Check sheet for the modelled part. Datum: model origin and axes. Units: mm. Face numbers are marked on the shaded views. A direction names the side the tool comes from. Coordinates: 2 decimals unless noted, no trailing zeros. Loops run counter-clockwise (first coordinate to the right, second up) from the corner with the lowest first, then second, coordinate; pieces in that order, holes last. Notation, with made-up numbers: (20.25, 14) - (33.25, 14) arc R25 cw to (33.25, 33) - close; hole circle Ø1 at (-33.5, -8). An arc over 180 degrees is marked (long way). Write each question's results on one line, items separated by ' | '. Start each with the question number.
1. Cross-section at A-A (z = -13). Record the cut outline in (x, y), and give its area (3 significant figures).
2. Cross-section at B-B (y = -170.5). Record the cut outline in (x, z), and give its area (3 significant figures).
3. Tool access check on the marked faces 1 and 2. Record the directions out of +Z, -Z, +X, -X, +Y, -Y that give a thin tool (end or side, any length) a straight path to the whole face; none if there is none.
4. Thickness scan on line 1 (Y direction, x = 11, z = -2.5); line 2 (Z direction, x = -0.5, y = -24); line 3 (Z direction, x = 0.5, y = -146). Record the ranges inside material, lowest first. Write a range as [from, to].
5. Cross-section at D-D (y = -12.5). Record the cut outline in (x, z) (3 decimals), and give its area (3 significant figures).
6. Gauge pin test, flat ends, axial feed: P1, Ø1.9, axis at x = -1, y = -159, coming from the +Z side; P2, Ø12, axis at y = -153, z = 2.5, coming from the -X side; P3, Ø1.5, axis at x = 11.5, y = -89, coming from the -Z side. Record the tip position at first contact, or that the pin passes through.
7. Cross-section at C-C (x = 13). Record the cut outline in (y, z).
```python
from build123d import *

# Parameters (mm, degrees)
CUT_EXTRUDE1_DEPTH      = 286.633670547
CUT_EXTRUDE1_DEPTH_BACK = 286.633670547
CUT_EXTRUDE2_DEPTH      = 286.633670547
CUT_EXTRUDE2_DEPTH_BACK = 286.633670547
BOSS_EXTRUDE1_DEPTH     = 13.7
SKETCH7_W               = 0.1
SKETCH7_H               = 0.8


with BuildPart() as part:
    # Sketch1 → Revolve1 (revolve)
    with BuildSketch(Plane.XY):
        with BuildLine():
            Line((0, 0), (15.875, 0))
            Line((15.875, 0), (15.875, -95.25))
            Line((15.875, -95.25), (7.75, -95.25))
            ThreePointArc((7.75, -95.25), (6.710108543, -97.13103799), (6.35, -99.25))
            Line((6.35, -99.25), (6.35, -123.35))
            ThreePointArc((6.35, -123.35), (6.765423592, -125.271598049), (7.9375, -126.85))
            Line((7.9375, -126.85), (7.9375, -148.15))
            Line((7.9375, -148.15), (6.35, -148.15))
            Line((6.35, -148.15), (6.35, -192.25))
            ThreePointArc((6.35, -192.25), (4.060973326, -193.504085038), (3.15, -195.95))
            Line((3.15, -195.95), (3.15, -236.95))
            ThreePointArc((3.15, -236.95), (2.021186638, -237.921495537), (1.6, -239.35))
            Line((1.6, -239.35), (1.6, -284.75))
            Line((1.6, -284.75), (0, -284.75))
            Line((0, -284.75), (0, 0))
        make_face()
    revolve(axis=Axis((0, -284.75, 0), (0, 1, 0)))

    # Sketch3 → Cut-Extrude1 (cut, two sides: drawn at the far end of the back side and taken through both)
    with BuildSketch(Plane.XY.offset(-CUT_EXTRUDE1_DEPTH_BACK)):
        with BuildLine():
            Line((7.9375, -139.15), (7.9375, -126.85))
            ThreePointArc((7.9375, -126.85), (7.511434792, -126.425239776), (7.14375, -125.949045798))
            Line((7.14375, -125.949045798), (7.14375, -139.15))
            Line((7.14375, -139.15), (7.9375, -139.15))
        make_face()
        with BuildLine():
            Line((-7.14375, -139.15), (-7.14375, -125.949045798))
            ThreePointArc((-7.14375, -125.949045798), (-7.511434792, -126.425239776), (-7.9375, -126.85))
            Line((-7.9375, -126.85), (-7.9375, -139.15))
            Line((-7.9375, -139.15), (-7.14375, -139.15))
        make_face()
    extrude(amount=CUT_EXTRUDE1_DEPTH + CUT_EXTRUDE1_DEPTH_BACK, mode=Mode.SUBTRACT)

    # Sketch4 → Cut-Extrude2 (cut, two sides: drawn at the far end of the back side and taken through both)
    with BuildSketch(Plane(origin=(0, 0, 0), x_dir=(0, 0, -1), z_dir=(1, 0, 0)).offset(-CUT_EXTRUDE2_DEPTH_BACK)):
        with BuildLine():
            Line((6.35, -163.5805), (6.2245, -163.5805))
            ThreePointArc((6.2245, -163.5805), (5.729525253, -163.375474747), (5.5245, -162.8805))
            Line((5.5245, -162.8805), (5.5245, -154.8825))
            ThreePointArc((5.5245, -154.8825), (5.729525253, -154.387525253), (6.2245, -154.1825))
            Line((6.2245, -154.1825), (6.35, -154.1825))
            Line((6.35, -154.1825), (6.35, -163.5805))
        make_face()
        with BuildLine():
            Line((-5.5245, -162.8805), (-5.5245, -154.8825))
            ThreePointArc((-5.5245, -154.8825), (-5.729525253, -154.387525253), (-6.2245, -154.1825))
            Line((-6.2245, -154.1825), (-6.35, -154.1825))
            Line((-6.35, -154.1825), (-6.35, -163.5805))
            Line((-6.35, -163.5805), (-6.2245, -163.5805))
            ThreePointArc((-6.2245, -163.5805), (-5.729525253, -163.375474747), (-5.5245, -162.8805))
        make_face()
    extrude(amount=CUT_EXTRUDE2_DEPTH + CUT_EXTRUDE2_DEPTH_BACK, mode=Mode.SUBTRACT)

    # Sketch5 → Boss-Extrude1 (add)
    with BuildSketch(Plane(origin=(0, 0, 0), x_dir=(1, 0, 0), z_dir=(0, 1, 0))):
        Polygon((-4.33708409, 7.51205), (-8.674168179, 0), (-4.33708409, -7.51205), (4.33708409, -7.51205), (8.674168179, 0), (4.33708409, 7.51205), align=None)
    extrude(amount=BOSS_EXTRUDE1_DEPTH)

    # Sketch6 → Revolve2 (revolve)
    with BuildSketch(Plane.XY, mode=Mode.PRIVATE) as revolve2_sk:
        Polygon((7.35, 13.7), (0, 13.7), (0, 50.2), (5.65, 50.2), align=None)
    revolve(revolve2_sk.sketch.rotate(Axis((0, 13.7, 0), (0, 1, 0)), 90), axis=Axis((0, 13.7, 0), (0, 1, 0)))

    # Sketch7 → Dont Clamp Below (revolve)
    with BuildSketch(Plane.XY):
        with Locations((15.925, -87.25)):
            Rectangle(SKETCH7_W, SKETCH7_H)
    revolve(axis=Axis((0, -284.75, 0), (0, 1, 0)))


solid = part.part
```
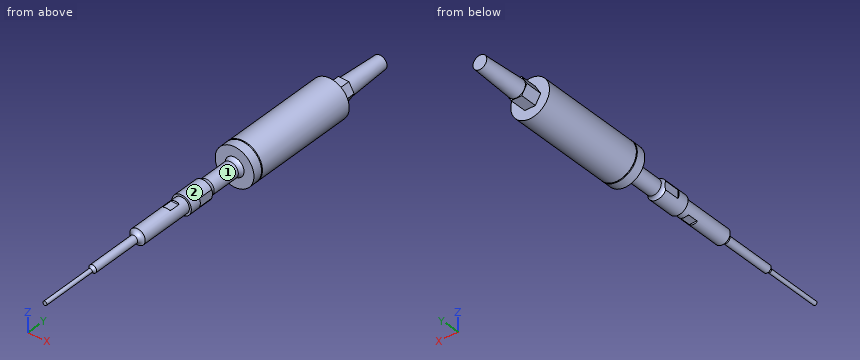
Established:
1) outline: (-9.28, -87.65) - (-9.11, -87.65) - (-9.11, -95.25) - (9.11, -95.25) - (9.11, -87.65) - (9.28, -87.65) - (9.28, -86.85) - (9.11, -86.85) - (9.11, 0) - (-9.11, 0) - (-9.11, -86.85) - (-9.28, -86.85) - close | area: 1,740 mm^2
2) outline: circle Ø12.7 at (0, 0) | area: 127 mm^2
3) face 1: none | face 2: -Y
4) line 1: [-95.25, 0] | line 2: [-15.87, 15.87] | line 3: [-7.92, 7.92]
5) outline: circle Ø31.75 at (0, 0) | area: 792 mm^2
6) P1: z = 5.52 | P2: x = -7.94 | P3: z = -11.68
7) outline: (-95.25, -9.11) - (-87.65, -9.11) - (-87.65, -9.28) - (-86.85, -9.28) - (-86.85, -9.11) - (0, -9.11) - (0, 9.11) - (-86.85, 9.11) - (-86.85, 9.28) - (-87.65, 9.28) - (-87.65, 9.11) - (-95.25, 9.11) - close
